Could you check a few things on this model? Use its own coordinates, in mm. Face numbers are marked on the shaded views. Coordinates: 2 decimals unless noted, no trailing zeros. Loops run counter-clockwise (first coordinate to the right, second up) from the corner with the lowest first, then second, coordinate; pieces in that order, holes last. Notation, with made-up numbers: (4, -36) - (61, -36) arc R25 ccw to (61, -6) - close; hole circle Ø10 at (65, 13.5). An arc over 180 degrees is marked (long way). One line per item, written item: value. Start each with the question number.
(1) If we mould it in two halves opening along X, with no side actions, what happens to the marked faces 1 and 2? For each: pulls with the +X half, pulls with the -X half, needs draft (parallel to the pull), parting line crosses it, or undercut.
(2) If we section it at A-A on y = -22.5: Write out the boundary of the cut face in (x, z) (3 decimals).
(3) If we section it at D-D on x = 36: Write out the boundary of the cut face in (y, z), then the cut area to 3 significant figures.
(4) If we section it at B-B on z = -93: Write out the boundary of the cut face in (x, y) (3 decimals).
(5) If I drill on line 1 along Z through (x, y) = (-60, -23.5); line 2 along X through (y, z) = (-28, -108) (3 decimals); line 3 along Y through (x, z) = (44.5, -7.5), over which ranges is the centre line in solid material (lowest first)? Write a range as from..to.
(6) If we section it at C-C on x = -57: Write out the boundary of the cut face in (y, z), then the cut area to 3 significant figures.
(7) I'm going to push flat-ended pins straight in: P1, Ø8, axis at x = -55.5, y = -11, coming from the +Z side; P2, Ø4, axis at y = -27, z = -32, coming from the -X side (3 decimals); P3, Ø3, axis at x = 38, z = 51.5, coming from the -Y side. Where does each tip first touch, or does it pass through?
```python
from build123d import *

# Parameters (mm, degrees)
F1_DEPTH = 19.05
F2_W     = 171.45
F2_H     = 215.9
F2_W_2   = 133.35
F2_H_2   = 177.8
F3_DEPTH = 12.7


with BuildPart() as f1:
    # F0 (on Front) → F1 (new body)
    with BuildSketch(Plane.XZ):
        with BuildLine():
            Line((-98.425, -133.35), (98.425, -133.35))
            Line((98.425, -133.35), (98.425, 77.419169))
            ThreePointArc((98.425, 77.419169), (80.719687, 109.600946), (44.059291, 111.872568))
            ThreePointArc((44.059291, 111.872568), (36.002014, 120.222357), (26.395227, 126.729917))
            ThreePointArc((26.395227, 126.729917), (6.848586, 145.313951), (-0.430385, 171.284205))
            ThreePointArc((-0.430385, 171.284205), (-7.4709, 145.248294), (-26.846302, 126.485796))
            ThreePointArc((-26.846302, 126.485796), (-36.197892, 120.056834), (-44.059291, 111.872568))
            ThreePointArc((-44.059291, 111.872568), (-80.719687, 109.600946), (-98.425, 77.419169))
            Line((-98.425, 77.419169), (-98.425, -133.35))
        make_face()
    extrude(amount=F1_DEPTH)

    # F2 (on face) → F3 (join)
    with BuildSketch(Plane.XZ.offset(19.05)):
        with Locations((0, -25.4)):
            Rectangle(F2_W, F2_H)
        with Locations((0, -25.4)):
            Rectangle(F2_W_2, F2_H_2, mode=Mode.SUBTRACT)
    extrude(amount=F3_DEPTH)


solid = f1.part
```
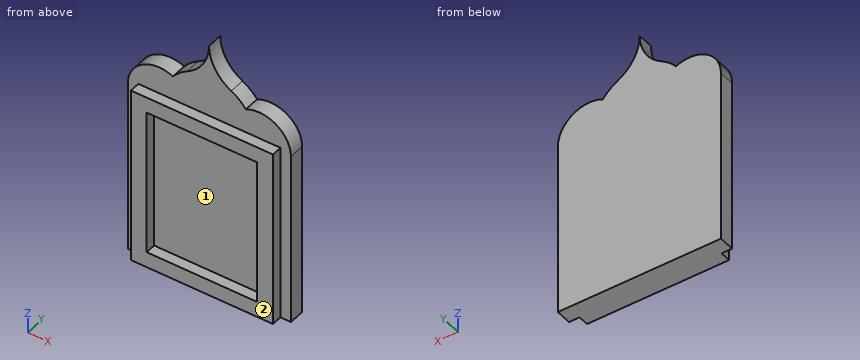
Values:
1. face 1: undercut
1. face 2: needs draft
2. outline: (-85.725, -133.35) - (85.725, -133.35) - (85.725, 82.55) - (-85.725, 82.55) - close; hole (-66.675, -114.3) - (66.675, -114.3) - (66.675, 63.5) - (-66.675, 63.5) - close
3. outline: (-31.75, -133.35) - (0, -133.35) - (0, 120.22) - (-19.05, 120.22) - (-19.05, 82.55) - (-31.75, 82.55) - (-31.75, 63.5) - (-19.05, 63.5) - (-19.05, -114.3) - (-31.75, -114.3) - close
3. area: 5,310 mm2
4. outline: (-98.425, -19.05) - (-85.725, -19.05) - (-85.725, -31.75) - (-66.675, -31.75) - (-66.675, -19.05) - (66.675, -19.05) - (66.675, -31.75) - (85.725, -31.75) - (85.725, -19.05) - (98.425, -19.05) - (98.425, 0) - (-98.425, 0) - close
5. line 1: z = -133.35..-114.3, 63.5..82.55
5. line 2: x = -85.725..-66.675, 66.675..85.725
5. line 3: y = -19.05..0
6. outline: (-31.75, -133.35) - (0, -133.35) - (0, 115.37) - (-19.05, 115.37) - (-19.05, 82.55) - (-31.75, 82.55) - (-31.75, 63.5) - (-19.05, 63.5) - (-19.05, -114.3) - (-31.75, -114.3) - close
6. area: 5,220 mm2
7. P1: stops at z = 115.51
7. P2: stops at x = -85.725
7. P3: stops at y = -19.05
